For this review, take the finished solid that the model builds, in its own axes (mm). Face numbers are marked on the shaded views. A direction names the side the tool comes from. Give positions to 0.01 mm unless a question says otherwise; leave off trailing zeros. Order: outer loops, then holes, each group sorted by start corner. A loop starts at its lowest first (then second) coordinate and runs counter-clockwise, first axis right, second up. Notation, with made-up numbers: (-4, 3.5) - (31, 3.5) arc R13 cw to (31, 24.5) - close; hole circle Ø11 at (69, 41). An arc over 180 degrees is marked (long way). One line per item, written item: value.
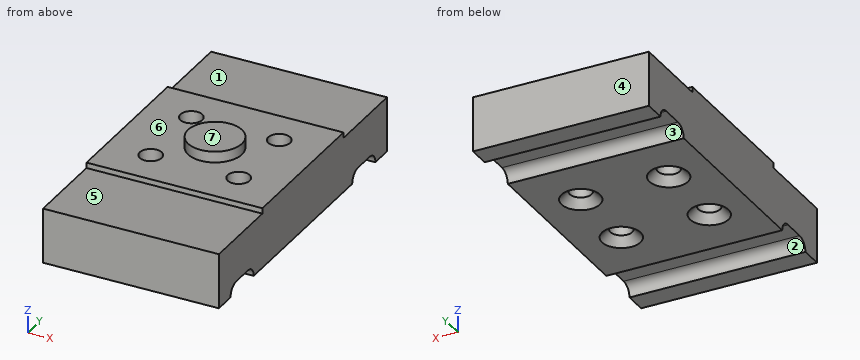
```python
from build123d import *

# Parameters (mm, degrees)
SKETCH_W      = 32
SKETCH_H      = 28
SKETCH_R      = 2
PAD_DEPTH     = 11
SKETCH001_R   = 4.9
PAD001_DEPTH  = 2
SKETCH002_W   = 32
SKETCH002_H   = 58
SKETCH002_W_2 = 25.648531
SKETCH002_H_2 = 22.342523
PAD002_DEPTH  = 10
POCKET_DEPTH  = 167.012111
CHAMFER_SIZE  = 1.5


with BuildPart() as part:
    # Sketch → Pad (new body)
    with BuildSketch(Plane.XY):
        Rectangle(SKETCH_W, SKETCH_H)
        with Locations((8, 7)):
            Circle(SKETCH_R, mode=Mode.SUBTRACT)
        with Locations((8, -7)):
            Circle(SKETCH_R, mode=Mode.SUBTRACT)
        with Locations((-8, -7)):
            Circle(SKETCH_R, mode=Mode.SUBTRACT)
        with Locations((-8, 7)):
            Circle(SKETCH_R, mode=Mode.SUBTRACT)
    extrude(amount=PAD_DEPTH)

    # Sketch001 (on Face10 of Pad) → Pad001 (join)
    with BuildSketch(Plane.XY.offset(11)):
        Circle(SKETCH001_R)
    extrude(amount=PAD001_DEPTH)

    # Sketch002 → Pad002 (join)
    with BuildSketch(Plane.XY):
        Rectangle(SKETCH002_W, SKETCH002_H)
        with Locations((-0.824266, 0.828739)):
            Rectangle(SKETCH002_W_2, SKETCH002_H_2, mode=Mode.SUBTRACT)
    extrude(amount=PAD002_DEPTH)

    # Sketch003 (on Face15 of Pad002) → Pocket (cut, through all)
    with BuildSketch(Plane(origin=(-16, 0, 0), x_dir=(0, -1, 0), z_dir=(-1, 0, 0))):
        with BuildLine():
            ThreePointArc((-23, 2), (-25, 0), (-23, -2))
            Line((-23, -2), (-19, -2))
            ThreePointArc((-19, -2), (-17, 0), (-19, 2))
            Line((-23, 2), (-19, 2))
        make_face()
    pocket = extrude(amount=-POCKET_DEPTH, mode=Mode.SUBTRACT)

    # Mirrored: Pocket across XZ
    add(pocket.mirror(Plane.XZ), mode=Mode.SUBTRACT)

    # Chamfer
    chamfer_edges = [part.edges().sort_by_distance(p)[0] for p in [
        (-10, 7, 0),
        (6, 7, 0),
        (6, -7, 0),
        (-10, -7, 0),
    ]]
    chamfer(chamfer_edges, length=CHAMFER_SIZE)


solid = part.part
```
(1) Machinability: for the marked faces 5, 6 and 7, which of the approach directions +Z, -Z, +X, -X, +Y, -Y give a long, thin tool a straight path to every point of the face, cutting with its end or side? Answer none if there is none.
Answers below:
face 5: +Z, +X, -X, -Y
face 6: +Z
face 7: +Z, +X, -X, +Y, -Y
(2) Draft analysis for pull direction Y (two halves, no side actions). For the marked faces 1, 2, 3 and 4, state which applies: pulls with the +Y half, pulls with the -Y half, needs draft (parallel to the pull), parting line crosses it, or undercut.
Answers below:
face 1: needs draft
face 2: undercut
face 3: undercut
face 4: pulls with the +Y half
(3) For P1, Ø4.5, axis at x = 8, y = -7, coming from the -Z side; P2, Ø5, axis at x = 8, y = 7, coming from the +Z side; P3, Ø4.5, axis at x = -7.5, y = 20, coming from the +Z side, all flat-tipped, find the tip position at first contact; note any pin that passes through.
Answers below:
P1: stops at z = 1.25
P2: stops at z = 11
P3: stops at z = 10
(4) Wall thickness on line 1 (Y direction, x = -8, z = 4); line 2 (Y direction, x = -6.5, z = 9.75); line 3 (Y direction, x = 7, z = 1.5): over which ranges is each line inside the solid? List them lowest first. Write a range as from..to.
Answers below:
line 1: y = -29..-9, -5..5, 9..29
line 2: y = -29..-8.32, -5.68..5.68, 8.32..29
line 3: y = -29..-24.32, -17.68..-8.73, -5.27..5.27, 8.73..17.68, 24.32..29
(5) Take a section at D-D (x = -14). Write out the cut boundary in (y, z).
Answers below:
outline: (-29, 0) - (-25, 0) arc R2 cw to (-23, 2) - (-19, 2) arc R2 cw to (-17, 0) - (17, 0) arc R2 cw to (19, 2) - (23, 2) arc R2 cw to (25, 0) - (29, 0) - (29, 10) - (14, 10) - (14, 11) - (-14, 11) - (-14, 10) - (-29, 10) - close
(6) Take a section at C-C (z = 3.25). Write out the cut boundary in (x, y).
Answers below:
outline: (-16, -29) - (16, -29) - (16, 29) - (-16, 29) - close; hole circle Ø4 at (-8, -7); hole circle Ø4 at (-8, 7); hole circle Ø4 at (8, -7); hole circle Ø4 at (8, 7)
(7) Take a section at A-A (y = 7). Write out the cut boundary in (x, z), then the cut area to 4 significant figures.
Answers below:
outline: (-16, 0) - (-11.5, 0) - (-10, 1.5) - (-10, 11) - (-16, 11) - close; (-6, 1.5) - (-4.5, 0) - (4.5, 0) - (6, 1.5) - (6, 11) - (-6, 11) - close; (10, 1.5) - (11.5, 0) - (16, 0) - (16, 11) - (10, 11) - close
area: 259.5 mm^2
(8) Take a section at B-B (x = 8). Write out the cut boundary in (y, z).
Answers below:
outline: (-29, 0) - (-25, 0) arc R2 cw to (-23, 2) - (-19, 2) arc R2 cw to (-17, 0) - (-10.5, 0) - (-9, 1.5) - (-9, 11) - (-14, 11) - (-14, 10) - (-29, 10) - close; (-5, 1.5) - (-3.5, 0) - (3.5, 0) - (5, 1.5) - (5, 11) - (-5, 11) - close; (9, 1.5) - (10.5, 0) - (17, 0) arc R2 cw to (19, 2) - (23, 2) arc R2 cw to (25, 0) - (29, 0) - (29, 10) - (14, 10) - (14, 11) - (9, 11) - close
